```python
from build123d import *

# Parameters (mm, degrees)
BOSS_EXTRUDE1_DEPTH = 228.6
SKETCH3_R           = 2.413
CUT_EXTRUDE1_DEPTH  = 1.905
LPATTERN1_COUNT     = 3
LPATTERN1_PITCH     = 76.2
CUT_EXTRUDE3_DEPTH  = 230.107436806
FILLET1_R           = 2.54
SKETCH5_W           = 114.3
SKETCH5_H           = 18.288
CUT_EXTRUDE4_DEPTH  = 230.107436806
FILLET2_R           = 1.27


with BuildPart() as part:
    # Sketch2 → Boss-Extrude1 (new, symmetric)
    with BuildSketch(Plane(origin=(0, 0, 0), x_dir=(0, 0, -1), z_dir=(1, 0, 0))):
        Polygon((0, 9.144), (-12.192, 9.144), (-12.192, 4.445), (-10.6045, 4.445), (-10.6045, 5.969), (-4.2545, 5.969), (-4.2545, 4.445), (-1.905, 4.445), (-1.905, -4.445), (-4.2545, -4.445), (-4.2545, -5.969), (-10.6045, -5.969), (-10.6045, -4.445), (-12.192, -4.445), (-12.192, -9.144), (0, -9.144), align=None)
    extrude(amount=BOSS_EXTRUDE1_DEPTH, both=True)

    # Sketch3 → Cut-Extrude1 (cut)
    with BuildSketch(Plane.XY.offset(1.905)):
        with Locations((38.1, 0)):
            Circle(SKETCH3_R)
    cut_extrude1 = extrude(amount=-CUT_EXTRUDE1_DEPTH, mode=Mode.SUBTRACT)

    # LPattern1: Cut-Extrude1 ×3
    with Locations(*[(i * LPATTERN1_PITCH, 0, 0) for i in range(1, LPATTERN1_COUNT)]):
        add(cut_extrude1, mode=Mode.SUBTRACT)

    # SurfaceCut1
    split(bisect_by=Plane(origin=(0, 0, 0), x_dir=(0, 0, -1), z_dir=(1, 0, 0)), keep=Keep.TOP)

    # Mirror1: part across plane


with BuildPart() as part_1:
    add(part.part)
    add(part.part.mirror(Plane(origin=(0, 0, 0), x_dir=(0, 0, 1), z_dir=(1, 0, 0))))

    # Sketch4 → Cut-Extrude3 (cut, through all)
    with BuildSketch(Plane.XY.offset(12.192)):
        Polygon((-209.55, -9.144), (-191.262, 9.144), (-228.6, 9.144), (-228.6, -9.144), align=None)
    extrude(amount=-CUT_EXTRUDE3_DEPTH, mode=Mode.SUBTRACT)

    # Fillet1
    # the kernel refuses this fillet: 2.54 mm, written as the material it takes off along each edge
    with BuildSketch(Plane(origin=(-209.55, -9.144, 27.522256121), x_dir=(0.7071067811865455, 0.7071067811865496, 0), z_dir=(0, 0, -1))) as fillet1_piece_1:
        with BuildLine():
            CenterArc((FILLET1_R * 2.41421356237, FILLET1_R), FILLET1_R, 135, 135)
            Line((FILLET1_R * 1.70710678119, FILLET1_R * 1.70710678119), (0, 0))
            Line((0, 0), (FILLET1_R * 2.41421356237, 0))
        make_face()
    extrude(amount=42.852512242, mode=Mode.SUBTRACT)

    # Sketch5 → Cut-Extrude4 (cut, through all)
    with BuildSketch(Plane.XY.offset(12.192)):
        with Locations((171.45, 0)):
            Rectangle(SKETCH5_W, SKETCH5_H)
    extrude(amount=-CUT_EXTRUDE4_DEPTH, mode=Mode.SUBTRACT)

    # Fillet2
    fillet2_edges = [part_1.edges().sort_by_distance(p)[0] for p in [
        (114.3, -9.144, 6.096),
        (114.3, 9.144, 6.096),
    ]]
    fillet(fillet2_edges, radius=FILLET2_R)


solid = part_1.part
```
Can you work these out from the model? Positions are in its coordinate system, mm. A direction names the side the tool comes from. Coordinates: 2 decimals unless noted, no trailing zeros. Loops run counter-clockwise (first coordinate to the right, second up) from the corner with the lowest first, then second, coordinate; pieces in that order, holes last. Notation, with made-up numbers: M 53.25,22.25 L 86.25,22.25 A19 ccw 86.25,52.25 Z; hole C -1,17.5 d11. An arc over 180 degrees is marked long. Put each result on its own line as item: value. Start each with the question number.
(1) Imagine slicing it at A-A on z = 7.5. List the corners of the cut face in (x, y) for me.
(2) Imagine slicing it at B-B on x = -154. List the corners of the cut face in (y, z) for me (1 decimal).
(3) Will this pin go through, and if not, where does the flat tip stop? pin 1 Ø4.5 at (x, y) = (-78, -1.5) entering from +Z (3 decimals).
(4) We'd pull the mould along Z, two halves only. Please class faces 1 (the face through (114.3, -6.4, 4.8)), 2 (the face through (-48, 0, 0)), 3 (the face through (-48, -5.969, 7)): +Z half, -Z half, draft (parallel to the pull), parting line (faces both ways), or undercut.
(5) Which directions (+Z, -Z, +X, -X, +Y, -Y) give clear straight access to the entire face, cutting with the end or side of a thin tool? Please do faces 4 (the face through (-42, 5.969, 7)), 5 (the face through (-48, 0, 1.905)), 6 (the face through (114.3, 6.3, 4.8)).
(6) I need wall thicknesses on probe 1 along Y at (x, z) = (-190.5, 1.55); probe 2 along Z at (x, y) = (-123, -5.75); probe 3 along Y at (x, z) = (-34, 11.75) (3 decimals). Which ranges of each line are inside material? Lowest first, please.
Worked answers:
1. outline: M -205.88,-5.97 A2.54 ccw -203.42,-9.14 L 113.03,-9.14 A1.27 ccw 114.3,-7.87 L 114.3,-5.97 Z; M -194.44,5.97 L 114.3,5.97 L 114.3,7.87 A1.27 ccw 113.03,9.14 L -191.26,9.14 Z
2. outline: M -9.1,0 L 9.1,0 L 9.1,12.2 L 4.4,12.2 L 4.4,10.6 L 6,10.6 L 6,4.3 L 4.4,4.3 L 4.4,1.9 L -4.4,1.9 L -4.4,4.3 L -6,4.3 L -6,10.6 L -4.4,10.6 L -4.4,12.2 L -9.1,12.2 Z
3. pin 1: stops at z = 1.905
4. face 1: draft
4. face 2: -Z half
4. face 3: undercut
5. face 4: +X, -X
5. face 5: +Z, +X, -X
5. face 6: +Z, -Z, +X, +Y, -Y
6. probe 1: y = -9.14 to -2.41, 2.41 to 9.14
6. probe 2: z = 0 to 4.25, 10.6 to 12.19
6. probe 3: y = -9.144 to -4.445, 4.445 to 9.144
